For this review, use the dimensioned drawing (mm, ordinates from the lowest corner) and the shaded views. A direction names the side the tool comes from. Round coordinates to 2 decimals unless told otherwise and drop trailing zeros. Loops run counter-clockwise (first coordinate to the right, second up) from the corner with the lowest first, then second, coordinate; pieces in that order, holes last. Notation, with made-up numbers: M 6.25,78 L 24.25,78 A17 ccw 24.25,101 Z; hole C 4,80.25 d10. An arc over 180 degrees is marked long. One line per item, written item: value. Start each with the question number.
Item 1: We need section C-C (y = 5.5). Write out the cut boundary in (x, z) (1 decimal).
Item 2: We need section D-D (z = 5.5). Write out the cut boundary in (x, y) (1 decimal).
Item 3: We need section B-B (x = 36.5). Write out the cut boundary in (y, z) (1 decimal).
Item 4: For line 1 along X through (y, z) = (5.75, 30) (1 decimal); line 2 along X through (y, z) = (5.25, 7) (1 decimal); line 3 along Y through (x, z) = (35.5, 3), list the stretches that pass through material, from the lowest coordinate up.
Item 5: Mouldability with a two-part tool opening along Z and no side actions: class the marked faces 1, 2 and 3 as released by +Z, released by -Z, zero draft, split by the parting line, or undercut.
Item 6: Clearance check with flat-ended pins moving along their axes: pin 1 (4 mm diameter, centred on y = 5, z = 44, fed in from +X); pin 2 (4 mm diameter, centred on x = 41.89, z = 51.04, fed in from +Y); pin 3 (5 mm diameter, centred on x = 50.5, z = 17.5, fed in from -Y). State where each tip first meets the part, or that it passes through.
Item 7: For the marked faces 4 and 5, list the 3-axis set-ups (+Z, -Z, +X, -X, +Y, -Y) from which the entire face can be reached by the end or side of a thin tool; tool diameter is ignored.
Item 8: We need section A-A (z = 26.5). Write out the cut boundary in (x, y) (1 decimal), then the cut area to 3 significant figures.
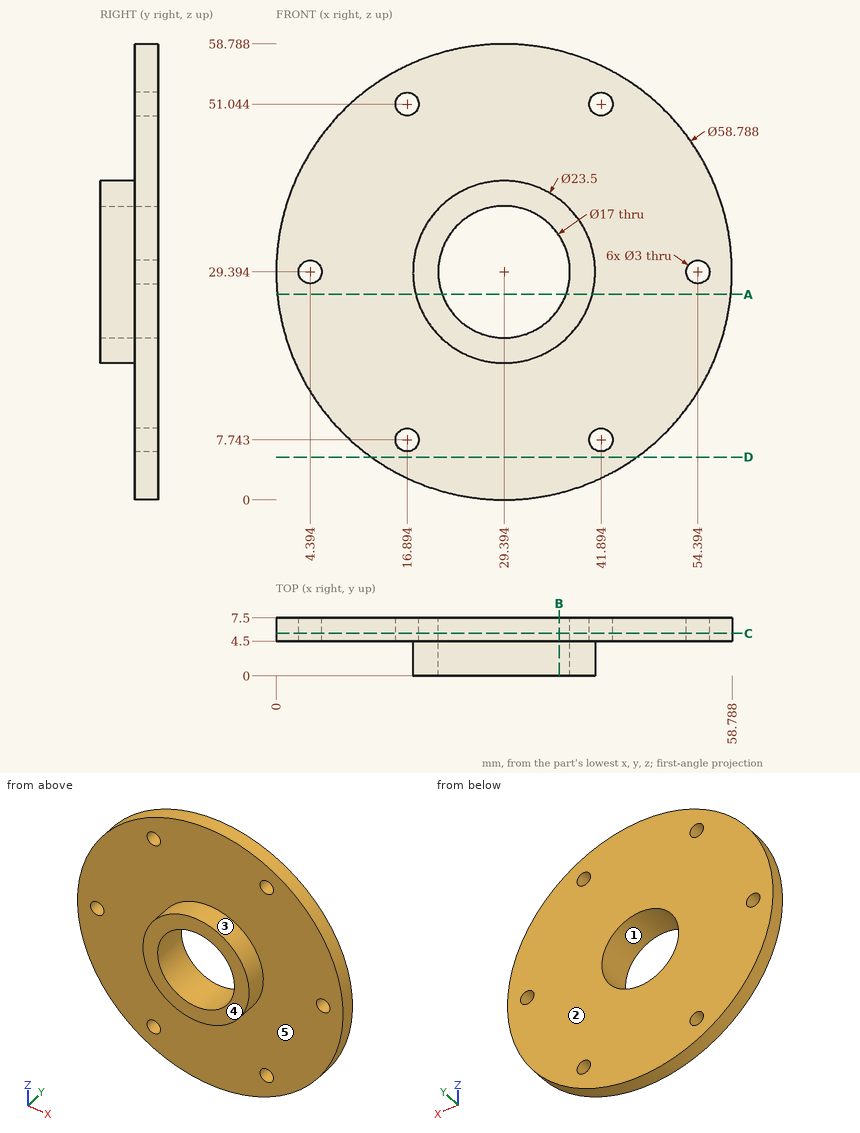
A:
1. outline: C 29.4,29.4 d58.8; hole C 4.4,29.4 d3; hole C 16.9,7.7 d3; hole C 16.9,51 d3; hole C 29.4,29.4 d17; hole C 41.9,7.7 d3; hole C 41.9,51 d3; hole C 54.4,29.4 d3
2. outline: M 12.3,4.5 L 46.5,4.5 L 46.5,7.5 L 12.3,7.5 Z
3. outline: M 0,20 L 4.5,20 L 4.5,0.9 L 7.5,0.9 L 7.5,24.7 L 0,24.7 Z; M 0,34.1 L 7.5,34.1 L 7.5,57.9 L 4.5,57.9 L 4.5,38.8 L 0,38.8 Z
4. line 1: 0 to 3, 5.8 to 20.9, 37.9 to 53, 55.8 to 58.8
4. line 2: 10.4 to 15.6, 18.2 to 40.6, 43.2 to 48.4
4. line 3: 4.5 to 7.5
5. face 1: undercut
5. face 2: zero draft
5. face 3: split by the parting line
6. pin 1: x = 55.95
6. pin 2: y = 7.5
6. pin 3: y = 4.5
7. face 4: +Z, -Z, +X, -X, -Y
7. face 5: -Y
8. outline: M 0.1,4.5 L 18,4.5 L 18,0 L 21.4,0 L 21.4,7.5 L 0.1,7.5 Z; M 37.4,0 L 40.8,0 L 40.8,4.5 L 58.6,4.5 L 58.6,7.5 L 37.4,7.5 Z
8. area: 158 mm2
